The listing builds one solid part. Answer for the finished solid, in the listing's coordinates (mm). A direction names the side the tool comes from. Coordinates: 2 decimals unless noted, no trailing zeros. Order: outer loops, then holes, each group sorted by start corner. A loop starts at its lowest first (then second) coordinate and runs counter-clockwise, first axis right, second up. Notation, with made-up numbers: (46, 76) -> (76, 76) arc R17 ccw to (76, 105) -> close; hole circle Ø5 at (29, -23). An arc over 180 degrees is marked (long way). Return JSON: item names as keys, results as strings.
```python
from build123d import *

# Parameters (mm, degrees)
F1_DEPTH = 5


with BuildPart() as f1:
    # F0 (on Front) → F1 (new body, symmetric)
    with BuildSketch(Plane.XZ):
        with BuildLine():
            Line((-2.95, 0), (0, 0))
            Line((0, 0), (0, 1.252587))
            ThreePointArc((0, 1.252587), (-1.520742, 1.440502), (-2.95, 1.992944))
            Line((-2.95, 1.992944), (-2.95, 0))
        make_face()
        with BuildLine():
            Line((0, 0), (2.95, 0))
            Line((2.95, 0), (2.95, 1.992944))
            ThreePointArc((2.95, 1.992944), (1.520742, 1.440502), (0, 1.252587))
            Line((0, 1.252587), (0, 0))
        make_face()
        with BuildLine():
            Line((2.95, 0), (15, 0))
            ThreePointArc((15, 0), (11.602801, 9.506577), (2.95, 14.707056))
            Line((2.95, 14.707056), (2.95, 13.007056))
            ThreePointArc((2.95, 13.007056), (6.247413, 7.5), (2.95, 1.992944))
            Line((2.95, 1.992944), (2.95, 0))
        make_face()
        with BuildLine():
            Line((-15, 0), (-2.95, 0))
            Line((-2.95, 0), (-2.95, 1.992944))
            ThreePointArc((-2.95, 1.992944), (-6.247413, 7.5), (-2.95, 13.007056))
            Line((-2.95, 13.007056), (-2.95, 13.857056))
            Line((-2.95, 13.857056), (-2.95, 14.707056))
            ThreePointArc((-2.95, 14.707056), (-11.602801, 9.506577), (-15, 0))
        make_face()
    extrude(amount=F1_DEPTH, both=True)


solid = f1.part
```
Item 1: Find the intervals of material crossed by probe 1 along X at (y, z) = (0.5, 10); probe 2 along Z at (x, y) = (5, 1.5); probe 3 along X at (y, z) = (3.5, 12.5), in increasing order.
Answer list:
{"probe 1": "-11.18 to -5.73, 5.73 to 11.18", "probe 2": "0 to 3.75, 11.25 to 14.14", "probe 3": "-8.29 to -3.75, 3.75 to 8.29"}
Item 2: The part is cut by section A-A on y = 1.5. Determine the outline of the cut face in (x, z).
Answer list:
{"outline": "(-15, 0) -> (15, 0) arc R15 ccw to (2.95, 14.71) -> (2.95, 13.01) arc R6.25 cw to (2.95, 1.99) arc R6.25 cw to (0, 1.25) arc R6.25 cw to (-2.95, 1.99) arc R6.25 cw to (-2.95, 13.01) -> (-2.95, 14.71) arc R15 ccw to start"}
Item 3: Flat-ended cylindrical pins translate along their axes: pin 1 (3 mm diameter, centred on x = -0.5, y = -4, fed in from +Z); pin 2 (1.4 mm diameter, centred on y = -2, z = 14, fed in from +X); pin 3 (1.5 mm diameter, centred on x = -1.5, y = 2, fed in from +Z). Find the tip coordinate at first contact, or state that the pin passes through.
Answer list:
{"pin 1": "z = 1.58", "pin 2": "x = 6.94", "pin 3": "z = 1.67"}
Item 4: Which of the six approach directions +Z, -Z, +X, -X, +Y, -Y give full straight-line access (tool end or side, diameter ignored) to faces 4 (the cylindrical face through (12, 0, 9)), 5 (the flat face through (2.95, 0, 14)), 6 (the cylindrical face through (6.247, -0.07, 7.594))?
Answer list:
{"face 4": "+Z, +X, +Y, -Y", "face 5": "+Z, +Y, -Y", "face 6": "+Y, -Y"}
Item 5: The part is cut by section C-C on z = 9.5. Determine the outline of the cut face in (x, y), plus the area to 3 significant figures.
Answer list:
{"outline": "(-11.61, -5) -> (-5.92, -5) -> (-5.92, 5) -> (-11.61, 5) -> close; (5.92, -5) -> (11.61, -5) -> (11.61, 5) -> (5.92, 5) -> close", "area": "114 mm2"}
Item 6: Determine the mould class of faces 1 (the flat face through (0, -5, 1)), 2 (the cylindrical face through (-6.247, -0.07, 7.406)), 3 (the flat face through (0, 0, 0)) for opening direction Z: pulls with the +Z half, pulls with the -Z half, needs draft (parallel to the pull), parting line crosses it, or undercut.
Answer list:
{"face 1": "needs draft", "face 2": "undercut", "face 3": "pulls with the -Z half"}
Item 7: The part is cut by section D-D on x = 9.5. Determine the outline of the cut face in (y, z).
Answer list:
{"outline": "(-5, 0) -> (5, 0) -> (5, 11.61) -> (-5, 11.61) -> close"}
Item 8: The part is cut by section B-B on z = 13.75. Determine the outline of the cut face in (x, y).
Answer list:
{"outline": "(-5.99, -5) -> (-2.95, -5) -> (-2.95, 5) -> (-5.99, 5) -> close; (2.95, -5) -> (5.99, -5) -> (5.99, 5) -> (2.95, 5) -> close"}
